Work out the finished part from the listing and answer in its coordinate system (mm). Face numbers are marked on the shaded views. A direction names the side the tool comes from. Round coordinates to 2 decimals unless told otherwise and drop trailing zeros. Write each loop counter-clockwise with the first axis right and the second up, starting at its lowest first coordinate (ties: lowest second). Pieces come first, ordered by that corner, then holes. Notation, with made-up numbers: (37.5, -9) - (69.5, -9) arc R8 cw to (69.5, 5) - close; hole circle Ø4 at (7, 62.25). An arc over 180 degrees is marked (long way). Answer as a JSON object with one key per item and string values.
```python
from build123d import *

# Parameters (mm, degrees)
F1_W         = 8.5
F1_H         = 20.4836754128
F2_DEPTH     = 4
F3_DEPTH     = 12
F4_DEPTH     = 4
F5_DEPTH     = 10
F6_T1_DEPTH  = 25
F7_T4_DEPTH  = 44.9785728407
F7_S6_R      = 3.75
F7_T7_DEPTH  = 24
F7_T11_DEPTH = 44.9785728407
F7_T16_DEPTH = 44.9785728407
F7_T21_DEPTH = 44.9785728407
F7_T26_DEPTH = 44.9785728407
F7_T31_DEPTH = 44.9785728407
F7_S33_R     = 3.75
F7_T34_DEPTH = 24


# Not quite as in the source:
# - a fillet or chamfer that OpenCascade refuses, or shapes differently, is made with other operations: its cross-section is extruded or revolved along the edge and cut away or added


with BuildPart() as f2:
    # F1 (on Top) → F2 (new body)
    with BuildSketch(Plane.XY):
        with Locations((4.25, -4.6106860973)):
            Rectangle(F1_W, F1_H)
        with Locations((-4.25, -4.6106860973)):
            Rectangle(F1_W, F1_H)
    extrude(amount=-F2_DEPTH)

    # F0 (on Top) → F3 (join)
    with BuildSketch(Plane.XY):
        with BuildLine():
            ThreePointArc((3.75, 0), (-2.6516504294, 2.6516504294), (0, -3.75))
            ThreePointArc((0, -3.75), (2.6516504294, -2.6516504294), (3.75, 0))
        make_face()
        with BuildLine():
            ThreePointArc((0, -2.25), (-1.5909902577, 1.5909902577), (2.25, 0))
            ThreePointArc((2.25, 0), (1.5909902577, -1.5909902577), (0, -2.25))
        make_face(mode=Mode.SUBTRACT)
        Polygon((7.5, -5.7213721946), (0, -5.7213721946), (-7.5, -5.7213721946), (-7.5, -12.7213721946), (7.5, -12.7213721946), align=None)
        Polygon((-4, -6.7213721946), (0, -6.7213721946), (4, -6.7213721946), (4, -11.7213721946), (-4, -11.7213721946), align=None, mode=Mode.SUBTRACT)
    extrude(amount=-F3_DEPTH)

    # F4 (cut): a face of the model
    f4_faces = [f2.faces().sort_by_distance(p)[0] for p in [
        (0, -9.2213721946, -4),
    ]]
    extrude(f4_faces, amount=-F4_DEPTH, mode=Mode.SUBTRACT)

    # F5 (add): a face of the model
    f5_faces = [f2.faces().sort_by_distance(p)[0] for p in [
        (0, 3.6439339828, -12),
    ]]
    extrude(f5_faces, amount=F5_DEPTH)

    # F6: fillet of radius 2 on 2 edges, made by hand

    # F6_s2 → F6_t1 (cut)
    with BuildSketch(Plane.YZ.offset(-12.5)):
        with BuildLine():
            ThreePointArc((-10.7213721946, -12), (-12.135585757, -11.4142135624), (-12.7213721946, -10))
            Line((-12.7213721946, -10), (-12.7213721946, -12))
            Line((-12.7213721946, -12), (-10.7213721946, -12))
        make_face()
        with BuildLine():
            ThreePointArc((-7.7213721946, -12), (-6.3071586322, -11.4142135624), (-5.7213721946, -10))
            Line((-5.7213721946, -10), (-5.7213721946, -12))
            Line((-5.7213721946, -12), (-7.7213721946, -12))
        make_face()
    extrude(amount=F6_T1_DEPTH, mode=Mode.SUBTRACT)

    # F7: fillet of radius 5 on 2 edges, made by hand


with BuildPart() as f7_tool2:
    # F7_s3 → F7_t4 (new body)
    with BuildSketch(Plane.XZ.offset(-17.8786003231)):
        with BuildLine():
            ThreePointArc((-3.6010205144, -4), (-6.7632981746, -2.8729833462), (-8.5, 0))
            Line((-8.5, 0), (-8.5, -4))
            Line((-8.5, -4), (-3.6010205144, -4))
        make_face()
    extrude(amount=F7_T4_DEPTH)

    split(bisect_by=Plane.XZ.offset(5.7213721946), keep=Keep.BOTTOM)

    # F7_s6 → F7_t7 (cut, symmetric)
    with BuildSketch(Plane.XY.offset(-2)):
        Circle(F7_S6_R)
    extrude(amount=F7_T7_DEPTH, both=True, mode=Mode.SUBTRACT)


with BuildPart() as f2_1:
    add(f2.part)

    # F7_t1: cut F7_tool2
    add(f7_tool2.part, mode=Mode.SUBTRACT)


with BuildPart() as f7_tool9:
    # F7_s10 → F7_t11 (new body)
    with BuildSketch(Plane.XZ.offset(-17.8786003231)):
        with BuildLine():
            ThreePointArc((-3.6010205144, -4), (-6.7632981746, -2.8729833462), (-8.5, 0))
            Line((-8.5, 0), (-8.5, -4))
            Line((-8.5, -4), (-3.6010205144, -4))
        make_face()
    extrude(amount=F7_T11_DEPTH)

    split(bisect_by=Plane.YZ.offset(-7.5), keep=Keep.BOTTOM)


with BuildPart() as f2_2:
    add(f2_1.part)

    # F7_t8: cut F7_tool9
    add(f7_tool9.part, mode=Mode.SUBTRACT)


with BuildPart() as f7_tool14:
    # F7_s15 → F7_t16 (new body)
    with BuildSketch(Plane.XZ.offset(-17.8786003231)):
        with BuildLine():
            ThreePointArc((-3.6010205144, -4), (-6.7632981746, -2.8729833462), (-8.5, 0))
            Line((-8.5, 0), (-8.5, -4))
            Line((-8.5, -4), (-3.6010205144, -4))
        make_face()
    extrude(amount=F7_T16_DEPTH)

    split(bisect_by=Plane.XZ.offset(12.7213721946), keep=Keep.TOP)


with BuildPart() as f2_3:
    add(f2_2.part)

    # F7_t13: cut F7_tool14
    add(f7_tool14.part, mode=Mode.SUBTRACT)


with BuildPart() as f7_tool19:
    # F7_s20 → F7_t21 (new body)
    with BuildSketch(Plane.XZ.offset(27.0999725176)):
        with BuildLine():
            ThreePointArc((8.5, 0), (6.7632981746, -2.8729833462), (3.6010205144, -4))
            Line((3.6010205144, -4), (8.5, -4))
            Line((8.5, -4), (8.5, 0))
        make_face()
    extrude(amount=-F7_T21_DEPTH)

    split(bisect_by=Plane.YZ.offset(7.5), keep=Keep.TOP)


with BuildPart() as f2_4:
    add(f2_3.part)

    # F7_t18: cut F7_tool19
    add(f7_tool19.part, mode=Mode.SUBTRACT)


with BuildPart() as f7_tool24:
    # F7_s25 → F7_t26 (new body)
    with BuildSketch(Plane.XZ.offset(27.0999725176)):
        with BuildLine():
            ThreePointArc((8.5, 0), (6.7632981746, -2.8729833462), (3.6010205144, -4))
            Line((3.6010205144, -4), (8.5, -4))
            Line((8.5, -4), (8.5, 0))
        make_face()
    extrude(amount=-F7_T26_DEPTH)

    split(bisect_by=Plane.XZ.offset(12.7213721946), keep=Keep.TOP)


with BuildPart() as f2_5:
    add(f2_4.part)

    # F7_t23: cut F7_tool24
    add(f7_tool24.part, mode=Mode.SUBTRACT)


with BuildPart() as f7_tool29:
    # F7_s30 → F7_t31 (new body)
    with BuildSketch(Plane.XZ.offset(27.0999725176)):
        with BuildLine():
            ThreePointArc((8.5, 0), (6.7632981746, -2.8729833462), (3.6010205144, -4))
            Line((3.6010205144, -4), (8.5, -4))
            Line((8.5, -4), (8.5, 0))
        make_face()
    extrude(amount=-F7_T31_DEPTH)

    split(bisect_by=Plane.XZ.offset(5.7213721946), keep=Keep.BOTTOM)

    # F7_s33 → F7_t34 (cut, symmetric)
    with BuildSketch(Plane.XY.offset(-2)):
        Circle(F7_S33_R)
    extrude(amount=F7_T34_DEPTH, both=True, mode=Mode.SUBTRACT)


with BuildPart() as f2_6:
    add(f2_5.part)

    # F7_t28: cut F7_tool29
    add(f7_tool29.part, mode=Mode.SUBTRACT)


solid = f2_6.part
```
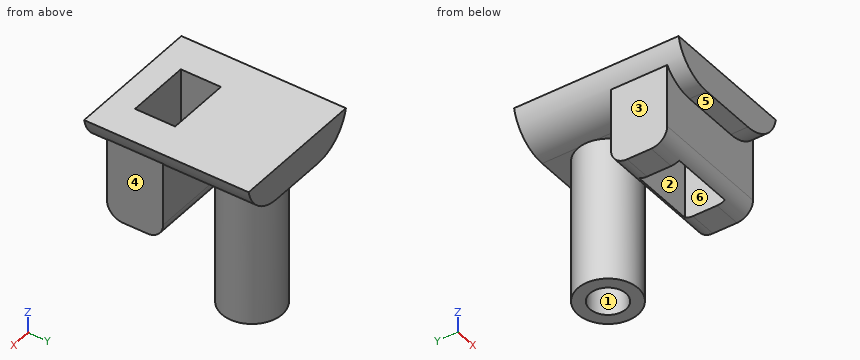
Item 1: Determine the mould class of the marked faces 4, 5 and 6 for opening direction X: pulls with the +X half, pulls with the -X half, needs draft (parallel to the pull), parting line crosses it, or undercut.
Results found:
{"face 4": "pulls with the +X half", "face 5": "needs draft", "face 6": "undercut"}
Item 2: Each of these flat-tipped pins is pushed along its axis until it touches: P1, Ø5, axis at x = 6.5, z = -8.5, coming from the +Y side; P2, Ø3.5, axis at x = 6, y = -9, coming from the -Z side; P3, Ø1, axis at x = -4.5, z = -10, coming from the -Y side. Where does it stop, or does it pass through?
Results found:
{"P1": "y = -5.72", "P2": "z = -12", "P3": "y = -12.72"}
Item 3: A cutting plane is placed at C-C (y = -8.5). Write down the section's boundary in (x, z).
Results found:
{"outline": "(-8.5, 0) arc R5 ccw to (-7.5, -2.13) - (-7.5, -12) - (-4, -12) - (-4, 0) - close; (4, -12) - (7.5, -12) - (7.5, -2.13) arc R5 ccw to (8.5, 0) - (4, 0) - close"}
Item 4: A cutting plane is placed at B-B (x = 0). Write down the section's boundary in (y, z), and give its area (3 significant figures).
Results found:
{"outline": "(-14.85, -4) - (-12.72, -4) - (-12.72, -10) arc R2 ccw to (-11.72, -11.73) - (-11.72, 0) - (-14.85, 0) - close; (-6.72, -11.73) arc R2 ccw to (-5.72, -10) - (-5.72, -4) - (-3.75, -4) - (-3.75, -22) - (-2.25, -22) - (-2.25, -4) - (2.25, -4) - (2.25, -22) - (3.75, -22) - (3.75, -4) - (5.63, -4) - (5.63, 0) - (-6.72, 0) - close", "area": "130 mm²"}
Item 5: Consider line 1 along X through (y, z) = (0, -7.5); line 2 along X through (y, z) = (-9.25, -3.75); line 3 along Y through (x, z) = (-5.25, -6.75). Determine where each line is inside the solid, lowest interval first.
Results found:
{"line 1": "-3.75 to -2.25, 2.25 to 3.75", "line 2": "-7.5 to -4, 4 to 7.5", "line 3": "-12.72 to -5.72"}
Item 6: A cutting plane is placed at D-D (y = 0). Write down the section's boundary in (x, z), and give its area (3 significant figures).
Results found:
{"outline": "(-8.5, 0) arc R5 ccw to (-3.75, -4) - (-3.75, -22) - (-2.25, -22) - (-2.25, -4) - (2.25, -4) - (2.25, -22) - (3.75, -22) - (3.75, -4) arc R5 ccw to (8.5, 0) - close", "area": "112 mm²"}
Item 7: A cutting plane is placed at A-A (z = -4.75). Write down the section's boundary in (x, y).
Results found:
{"outline": "(-7.5, -12.72) - (7.5, -12.72) - (7.5, -5.72) - (-7.5, -5.72) - close; circle Ø7.5 at (0, 0); hole (-4, -11.72) - (4, -11.72) - (4, -6.72) - (-4, -6.72) - close; hole circle Ø4.5 at (0, 0)"}
Item 8: For the marked faces 1, 2 and 3, determine the directions among +Z, -Z, +X, -X, +Y, -Y from which every point of the face is accessible in a straight line to the end or side of a thin tool.
Results found:
{"face 1": "-Z", "face 2": "+Z, -Z", "face 3": "-Z, -X, +Y, -Y"}
